from build123d import *

# Parameters (mm, degrees)
F0_R     = 85
F2_R     = 0.5
F4_R     = 105.9677495378
F5_DEPTH = 1


# Not quite as in the source:
# - a fillet or chamfer that OpenCascade refuses, or shapes differently, is made with other operations: its cross-section is extruded or revolved along the edge and cut away or added


with BuildPart() as f3:
    # F0 (on Top) → F3 section 0
    with BuildSketch(Plane.XY):
        Circle(F0_R)
    # F2 (on offset) → F3 section 1
    with BuildSketch(Plane.XY.offset(800)):
        Circle(F2_R)
    loft()

    # F4 (on Top) → F5 (join)
    with BuildSketch(Plane.XY):
        Circle(F4_R)
    extrude(amount=F5_DEPTH)

    # F6: fillet of radius 50 on 1 edges, made by hand


with BuildPart() as f6_tool2:
    # F6_s3 → F6_t4 (revolve)
    with BuildSketch(Plane.XZ):
        with BuildLine():
            ThreePointArc((105.9675526746, 0.9996517976), (88.7718520485, 17.0936422209), (80.851270192, 39.2741072932))
            Line((80.851270192, 39.2741072932), (75.8787755878, 38.7488875506))
            ThreePointArc((75.8787755878, 38.7488875506), (77.9005268853, 19.6118549121), (79.9218803957, 0.4747802574))
            Line((79.9218803957, 0.4747802574), (84.894375, -4.0001558343))
            ThreePointArc((84.894375, -4.0001558343), (95.4309638373, -4.0001558343), (103.5066863186, -3.3530134945))
            Line((103.5066863186, -3.3530134945), (105.9675526746, 0.9996517976))
        make_face()
    revolve(axis=Axis((0, 0, 1), (0, 0, 1)))

    split(bisect_by=Plane.XY, keep=Keep.TOP)


with BuildPart() as f3_1:
    add(f3.part)

    # F6_t1: union F6_tool2
    add(f6_tool2.part)


solid = f3_1.part
The listing builds one solid part. Answer for the finished solid, in the listing's coordinates (mm). Give positions to 0.01 mm unless a question says otherwise; leave off trailing zeros. Loops run counter-clockwise (first coordinate to the right, second up) from the corner with the lowest first, then second, coordinate; pieces in that order, holes last.
Item 1: Find the intervals of material crossed by line 1 along Z through (x, y) = (-78.5, 39.5); line 2 along Z through (x, y) = (-63.5, -59); line 3 along Y through (x, z) = (-52, 91), in increasing order.
Derived:
line 1: z = 0 to 18.51
line 2: z = 0 to 20.58
line 3: y = -54.58 to 54.58
Item 2: A cutting plane is placed at B-B (z = 186). Give the vertices of the cut face in (x, y), then the cut area to 3 significant figures.
Derived:
outline: circle Ø130.71 at (0, 0)
area: 13,400 mm2
Item 3: Each of these flat-tipped pins is pushed along its axis until it touches: pin 1 Ø12 at (x, z) = (-20.5, 565.5) entering from +Y; pin 2 Ø12 at (x, z) = (29.5, 501) entering from -Y; pin 3 Ø3 at (x, z) = (4.5, 535.5) entering from +Y. Where does it stop, or does it pass through?
Derived:
pin 1: stops at y = 20.77
pin 2: stops at y = -21.91
pin 3: stops at y = 28.34
Item 4: A cutting plane is placed at A-A (z = 344). Give the vertices of the cut face in (x, y) (3 decimals).
Derived:
outline: circle Ø97.33 at (0, 0)
